```python
from build123d import *

# Parameters (mm, degrees)
SKETCH3_W           = 12.7
SKETCH3_H           = 35
SKETCH3_W_2         = 40
SKETCH3_H_2         = 12.7
BOSS_EXTRUDE1_DEPTH = 12.7
SKETCH4_W           = 40
SKETCH4_H           = 12.7
CUT_EXTRUDE1_DEPTH  = 12.7


with BuildPart() as part:
    # Sketch3 → Boss-Extrude1 (new body)
    with BuildSketch(Plane.XY):
        Polygon((127.7, 60), (-127.7, 60), (-127.7, -25), (-127.7, -60), (-20, -60), (20, -60), (127.7, -60), (127.7, -25), align=None)
        with Locations((-134.05, -42.5)):
            Rectangle(SKETCH3_W, SKETCH3_H)
        with Locations((134.05, -42.5)):
            Rectangle(SKETCH3_W, SKETCH3_H)
        with Locations((0, -66.35)):
            Rectangle(SKETCH3_W_2, SKETCH3_H_2)
    extrude(amount=BOSS_EXTRUDE1_DEPTH)

    # Sketch4 → Cut-Extrude1 (cut)
    with BuildSketch(Plane.XY.offset(12.7)):
        with Locations((0, 53.65)):
            Rectangle(SKETCH4_W, SKETCH4_H)
    extrude(amount=-CUT_EXTRUDE1_DEPTH, mode=Mode.SUBTRACT)


solid = part.part
```
Verification items for the finished model (mm, model axes). A direction names the side the tool comes from. Round coordinates to 2 decimals unless told otherwise and drop trailing zeros. Order: outer loops, then holes, each group sorted by start corner. A loop starts at its lowest first (then second) coordinate and runs counter-clockwise, first axis right, second up.
1) Depth check by flat-ended pin: pin 1 (6.5 mm diameter, centred on y = 0.5, z = 7.5, fed in from -X); pin 2 (5 mm diameter, centred on y = 1, z = 4.5, fed in from +X); pin 3 (4 mm diameter, centred on x = 1, z = 5, fed in from +Y). Enter the tip coordinate at first touch or a pass-through.
Geometry says:
pin 1: stops at x = -127.7
pin 2: stops at x = 127.7
pin 3: stops at y = 47.3
2) Cross-section at A-A, the plane z = 10. Record the cut outline in (x, y).
Geometry says:
outline: (-140.4, -60) - (-20, -60) - (-20, -72.7) - (20, -72.7) - (20, -60) - (140.4, -60) - (140.4, -25) - (127.7, -25) - (127.7, 60) - (20, 60) - (20, 47.3) - (-20, 47.3) - (-20, 60) - (-127.7, 60) - (-127.7, -25) - (-140.4, -25) - close
3) Cross-section at B-B, the plane x = 103.5. Record the cut outline in (y, z).
Geometry says:
outline: (-60, 0) - (60, 0) - (60, 12.7) - (-60, 12.7) - close
4) Tool access check on faces 4 (the flat face through (-20, -66, 6)), 5 (the flat face through (20, -66, 6)), 6 (the flat face through (0, 47.3, 6)), 7 (the flat face through (-134, -25, 6)), 8 (the flat face through (134, -25, 6)). Record the directions out of +Z, -Z, +X, -X, +Y, -Y that give a thin tool (end or side, any length) a straight path to the whole face; none if there is none.
Geometry says:
face 4: +Z, -Z, -X, -Y
face 5: +Z, -Z, +X, -Y
face 6: +Z, -Z, +Y
face 7: +Z, -Z, -X, +Y
face 8: +Z, -Z, +X, +Y
5) Draft check along X on faces 1 (the flat face through (79, -60, 6)), 2 (the flat face through (-20, 54, 6)), 3 (the flat face through (127.7, 17, 6)). Enter one of: +X half, -X half, draft (parallel to the pull), parting line (faces both ways), or undercut.
Geometry says:
face 1: draft
face 2: undercut
face 3: +X half
6) Material ranges on line 1 (X direction, y = 49, z = 4); line 2 (Y direction, x = -47, z = 3.5); line 3 (X direction, y = -67, z = 2.5), recorded low to high.
Geometry says:
line 1: x = -127.7 to -20, 20 to 127.7
line 2: y = -60 to 60
line 3: x = -20 to 20
7) Cross-section at C-C, the plane y = 0.5. Record the cut outline in (x, z).
Geometry says:
outline: (-127.7, 0) - (127.7, 0) - (127.7, 12.7) - (-127.7, 12.7) - close
